Work out the finished part from the listing and answer in its coordinate system (mm). A direction names the side the tool comes from. Give positions to 0.01 mm unless a question says otherwise; leave off trailing zeros. Loops run counter-clockwise (first coordinate to the right, second up) from the corner with the lowest first, then second, coordinate; pieces in that order, holes last. Notation, with made-up numbers: (35.5, 86.25) - (61.5, 86.25) arc R35 ccw to (61.5, 121.25) - close; hole circle Ø4 at (42, 77). An arc over 180 degrees is marked (long way). Use CSV: the item, a comma, the result in double quotes.
from build123d import *

# Parameters (mm, degrees)
SKETCH2_W           = 5
SKETCH2_H           = 5
FILLET1_R           = 2.5
SKETCH3_W           = 5
SKETCH3_H           = 29.5
BOSS_EXTRUDE1_DEPTH = 2.5
SKETCH4_W           = 10
SKETCH4_H           = 10
BOSS_EXTRUDE2_DEPTH = 6


with BuildPart() as part:
    # Sweep3: sweep along a path in Sketch1
    with BuildLine(Plane(origin=(0, 0, 0), x_dir=(1, 0, 0), z_dir=(0, 1, 0))) as sweep3_path:
        Line((0, 0), (50, 0))
        ThreePointArc((50, 0), (80.614674589, 6.089637399), (106.568542495, 23.431457505))
        Line((106.568542495, 23.431457505), (141.923881554, 58.786796564))
    # Sketch2 → Sweep3 (sweep)
    with BuildSketch(Plane(origin=(0, 0, 0), x_dir=(0, 0, -1), z_dir=(1, 0, 0))):
        Rectangle(SKETCH2_W, SKETCH2_H)
    sweep(path=sweep3_path.line)

    # Fillet1
    fillet1_edges = [part.edges().sort_by_distance(p)[0] for p in [
        (122.478445072, -2.5, -42.876893988),
        (79.657966008, -2.5, -8.39933623),
        (122.478445072, 2.5, -42.876893988),
        (79.657966008, 2.5, -8.39933623),
        (25, -2.5, -2.5),
        (25, 2.5, -2.5),
    ]]
    fillet(fillet1_edges, radius=FILLET1_R - 0.0001)  # a hair under: the kernel refuses the full size

    # Sketch3 → Boss-Extrude1 (add, symmetric)
    with BuildSketch(Plane(origin=(0, 0, 0), x_dir=(1, 0, 0), z_dir=(0, 1, 0))):
        with Locations((2.5, -17.25)):
            Rectangle(SKETCH3_W, SKETCH3_H)
        Polygon((108.336309448, 21.663690552), (113.336309448, 26.663690552), (113.336309448, -32), (108.336309448, -32), align=None)
    extrude(amount=BOSS_EXTRUDE1_DEPTH, both=True)

    # Sketch4 → Boss-Extrude2 (add)
    with BuildSketch(Plane.XY.offset(32)):
        with Locations((2.5, -2.5)):
            Rectangle(SKETCH4_W, SKETCH4_H)
        with Locations((110.836309448, -2.5)):
            Rectangle(SKETCH4_W, SKETCH4_H)
    extrude(amount=-BOSS_EXTRUDE2_DEPTH)


solid = part.part
Item 1: For faces 1 (the flat face through (2, -4, 26)), 2 (the flat face through (7.5, -3, 29)), 3 (the flat face through (115.836, -3, 29)), 4 (the flat face through (113.336, 0, -1)), determine the directions among +Z, -Z, +X, -X, +Y, -Y from which every point of the face is accessible in a straight line to the end or side of a thin tool.
Determined:
face 1,"-Y"
face 2,"+Z, +Y, -Y"
face 3,"+Z, +X, +Y, -Y"
face 4,"+X, +Y, -Y"
Item 2: Given P1, Ø1, axis at y = -2.5, z = 6.5, coming from the +X side; P2, Ø5, axis at x = 4.5, y = -4, coming from the -Z side; P3, Ø5, axis at y = -2, z = -46, coming from the +X side, each flat-ended and moving along its own axis, determine where each tip first touches the part or whether it passes through.
Determined:
P1,"stops at x = 113.34"
P2,"stops at z = -2"
P3,"stops at x = 135.17"
Item 3: The mould has two halves that part along Z. Classify faces 5 (the cylindrical face through (123.26, -1.79, -42.59)), 6 (the flat face through (2, -2, 32)), 7 (the flat face through (105.836, -3, 29)), 8 (the flat face through (108.336, 0, 3)): pulls with the +Z half, pulls with the -Z half, needs draft (parallel to the pull), parting line crosses it, or undercut.
Determined:
face 5,"pulls with the -Z half"
face 6,"pulls with the +Z half"
face 7,"needs draft"
face 8,"undercut"
Item 4: A cutting plane is placed at A-A on z = 22. Determine the outline of the cut face in (x, y), and give its area (3 significant figures).
Determined:
outline,"(0, -2.5) - (5, -2.5) - (5, 2.5) - (0, 2.5) - close; (108.34, -2.5) - (113.34, -2.5) - (113.34, 2.5) - (108.34, 2.5) - close"
area,"50.0 mm²"
Item 5: Find the intervals of material crossed by line 1 (X direction, y = -2, z = 6); line 2 (Z direction, x = 5.5, y = 0); line 3 (Z direction, x = 113.5, y = -2), in increasing order.
Determined:
line 1,"x = 0 to 5, 108.34 to 113.34"
line 2,"z = -2.5 to 2.5, 26 to 32"
line 3,"z = -32.48 to -26.83, 26 to 32"
Item 6: A cutting plane is placed at B-B on y = -4.5. Determine the outline of the cut face in (x, z).
Determined:
outline,"(-2.5, 26) - (7.5, 26) - (7.5, 32) - (-2.5, 32) - close; (105.84, 26) - (115.84, 26) - (115.84, 32) - (105.84, 32) - close"
